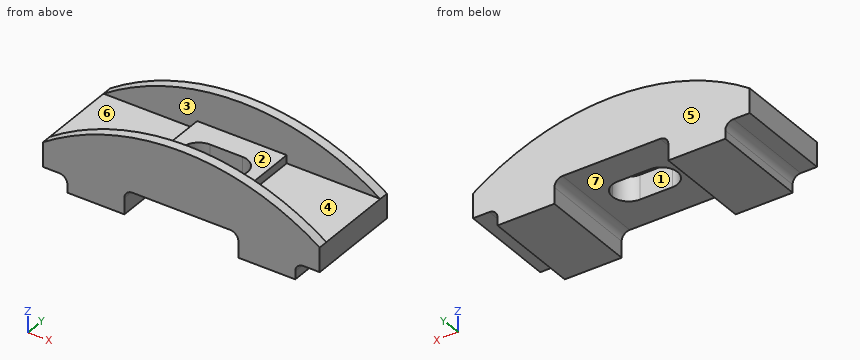
from build123d import *

# Parameters (mm, degrees)
F0_W      = 1700
F0_H      = 600
F1_DEPTH  = 250
F2_W      = 550
F2_H      = 480
F3_DEPTH  = 50
F5_DEPTH  = 300.001
F7_DEPTH  = 600.001
F9_DEPTH  = 600.001
F12_DEPTH = 60
F13_DEPTH = 60


with BuildPart() as f1:
    # F0 (on Top) → F1 (new body)
    with BuildSketch(Plane.XY):
        Rectangle(F0_W, F0_H)
    extrude(amount=F1_DEPTH)

    # F2 (on face) → F3 (join)
    with BuildSketch(Plane.XY.offset(250)):
        Rectangle(F2_W, F2_H)
    extrude(amount=F3_DEPTH)

    # F4 (on face) → F5 (cut, through all)
    with BuildSketch(Plane.XY.offset(300)):
        with BuildLine():
            ThreePointArc((-100, 100), (-200, 0), (-100, -100))
            Line((-100, -100), (-100, 100))
        make_face()
        with BuildLine():
            Line((-100, 100), (-100, -100))
            ThreePointArc((-100, -100), (-29.2893218813, -70.7106781187), (0, 0))
            ThreePointArc((0, 0), (-29.2893218813, 70.7106781187), (-100, 100))
        make_face()
        with BuildLine():
            ThreePointArc((0, 0), (29.2893218813, -70.7106781187), (100, -100))
            Line((100, -100), (100, 100))
            ThreePointArc((100, 100), (29.2893218813, 70.7106781187), (0, 0))
        make_face()
        with BuildLine():
            Line((100, 100), (100, -100))
            ThreePointArc((100, -100), (170.7106781187, -70.7106781187), (200, 0))
            ThreePointArc((200, 0), (170.7106781187, 70.7106781187), (100, 100))
        make_face()
        with BuildLine():
            ThreePointArc((0, 0), (29.2893218813, 70.7106781187), (100, 100))
            Line((100, 100), (-100, 100))
            ThreePointArc((-100, 100), (-29.2893218813, 70.7106781187), (0, 0))
        make_face()
        with BuildLine():
            Line((-100, -100), (100, -100))
            ThreePointArc((100, -100), (29.2893218813, -70.7106781187), (0, 0))
            ThreePointArc((0, 0), (-29.2893218813, -70.7106781187), (-100, -100))
        make_face()
    extrude(amount=-F5_DEPTH, mode=Mode.SUBTRACT)

    # F6 (on face) → F7 (cut, through all)
    with BuildSketch(Plane.XZ.offset(300)):
        with BuildLine():
            Line((-350, 0), (0, 0))
            Line((0, 0), (0, 150))
            Line((0, 150), (-300, 150))
            ThreePointArc((-300, 150), (-335.3553390593, 135.3553390593), (-350, 100))
            Line((-350, 100), (-350, 0))
        make_face()
        with BuildLine():
            Line((0, 150), (0, 0))
            Line((0, 0), (350, 0))
            Line((350, 0), (350, 100))
            ThreePointArc((350, 100), (335.3553390593, 135.3553390593), (300, 150))
            Line((300, 150), (0, 150))
        make_face()
    extrude(amount=-F7_DEPTH, mode=Mode.SUBTRACT)

    # F8 (on face) → F9 (cut, through all)
    with BuildSketch(Plane.XZ.offset(300)):
        with BuildLine():
            Line((850, 0), (850, 100))
            Line((850, 100), (750, 100))
            ThreePointArc((750, 100), (714.6446609407, 85.3553390593), (700, 50))
            Line((700, 50), (700, 0))
            Line((700, 0), (850, 0))
        make_face()
        with BuildLine():
            Line((-850, 100), (-850, 0))
            Line((-850, 0), (-700, 0))
            Line((-700, 0), (-700, 50))
            ThreePointArc((-700, 50), (-714.6446609407, 85.3553390593), (-750, 100))
            Line((-750, 100), (-850, 100))
        make_face()
    extrude(amount=-F9_DEPTH, mode=Mode.SUBTRACT)

    # F11 (on face) → F12 (join)
    with BuildSketch(Plane(origin=(0, 300, 0), x_dir=(-1, 0, 0), z_dir=(0, 1, 0))):
        with BuildLine():
            Line((-850, 250), (850, 250))
            ThreePointArc((850, 250), (0, 514.0792905692), (-850, 250))
        make_face()
    extrude(amount=-F12_DEPTH)

    # F10 (on face) → F13 (join)
    with BuildSketch(Plane.XZ.offset(300)):
        with BuildLine():
            Line((-850, 250), (850, 250))
            ThreePointArc((850, 250), (0, 514.0792905692), (-850, 250))
        make_face()
    extrude(amount=-F13_DEPTH)


solid = f1.part
The listing builds one solid part. Answer for the finished solid, in the listing's coordinates (mm). Face numbers are marked on the shaded views. A direction names the side the tool comes from. Give positions to 0.01 mm unless a question says otherwise; leave off trailing zeros. Loops run counter-clockwise (first coordinate to the right, second up) from the corner with the lowest first, then second, coordinate; pieces in that order, holes last.
Item 1: Determine the mould class of the marked faces 5, 6 and 7 for opening direction Y: +Y half, -Y half, draft (parallel to the pull), parting line (faces both ways), or undercut.
Derived:
face 5: +Y half
face 6: undercut
face 7: draft
Item 2: A cutting plane is placed at A-A (x = 39.5). Give the vertices of the cut face in (y, z).
Derived:
outline: (-300, 150) - (-100, 150) - (-100, 300) - (-240, 300) - (-240, 513.56) - (-300, 513.56) - close; (100, 150) - (300, 150) - (300, 513.56) - (240, 513.56) - (240, 300) - (100, 300) - close
Item 3: A cutting plane is placed at B-B (z = 405.5). Give the vertices of the cut face in (x, y), then the cut area to 3 significant figures.
Derived:
outline: (-560.31, -300) - (560.31, -300) - (560.31, -240) - (-560.31, -240) - close; (-560.31, 240) - (560.31, 240) - (560.31, 300) - (-560.31, 300) - close
area: 134,000 mm2
Item 4: A cutting plane is placed at C-C (y = 191). Give the vertices of the cut face in (x, z), then the cut area to 3 significant figures.
Derived:
outline: (-850, 100) - (-750, 100) arc R50 cw to (-700, 50) - (-700, 0) - (-350, 0) - (-350, 100) arc R50 cw to (-300, 150) - (300, 150) arc R50 cw to (350, 100) - (350, 0) - (700, 0) - (700, 50) arc R50 cw to (750, 100) - (850, 100) - (850, 250) - (275, 250) - (275, 300) - (-275, 300) - (-275, 250) - (-850, 250) - close
area: 320,000 mm2
Item 5: A tool of negligible diameter and unlimited length cuts with its end or side. For the marked faces 1, 2, 3 and 4, from which of +Z, -Z, +X, -X, +Y, -Y can it reach the whole face along a straight path? Write none if from no direction.
Derived:
face 1: +Z, -Z
face 2: +Z, +X, -X
face 3: +Z
face 4: +Z, +X
Item 6: Find the intervals of material crossed by line 1 along Y through (x, z) = (-447.5, 336.5); line 2 along X through (y, z) = (-223.5, 44); line 3 along Z through (x, y) = (-501.5, -51.5), in increasing order.
Derived:
line 1: y = -300 to -240, 240 to 300
line 2: x = -700 to -350, 350 to 700
line 3: z = 0 to 250
Item 7: Each of these flat-tipped pins is pushed along its axis until it touches: pin 1 Ø25 at (y, z) = (-5.5, 24) entering from -X; pin 2 Ø15 at (y, z) = (-92.5, 14) entering from +X; pin 3 Ø10 at (x, y) = (384.5, 23) entering from +Z. Where does it stop, or does it pass through?
Derived:
pin 1: stops at x = -700
pin 2: stops at x = 700
pin 3: stops at z = 250
Item 8: A cutting plane is placed at D-D (x = -579). Give the vertices of the cut face in (y, z), then the cut area to 3 significant figures.
Derived:
outline: (-300, 0) - (300, 0) - (300, 397.83) - (240, 397.83) - (240, 250) - (-240, 250) - (-240, 397.83) - (-300, 397.83) - close
area: 168,000 mm2
